from build123d import *

# Parameters (mm, degrees)
SKETCH1_R               = 7.5565
BOSS_EXTRUDE1_DEPTH     = 15.875
BOSS_EXTRUDE2_START     = 3.175
SKETCH2_R               = 7.5565
SKETCH2_R_2             = 3.3782
BOSS_EXTRUDE2_DEPTH     = 3.175
CUT_EXTRUDE1_DEPTH      = 20.136797263
CUT_EXTRUDE1_DEPTH_BACK = 20.136797263
SKETCH3_W               = 1.979009817
SKETCH3_H               = 3.81
SKETCH3_W_2             = 2.256055482


with BuildPart() as part:
    # Sketch1 → Boss-Extrude1 (new body)
    with BuildSketch(Plane(origin=(0, 0, 0), x_dir=(1, 0, 0), z_dir=(0, 1, 0))):
        with Locations(Location((0, 0, 0), (0, 0, 270))):
            Circle(SKETCH1_R)
        Polygon((-3.207902433, 5.55625), (-6.415804866, 0), (-3.207902433, -5.55625), (3.207902433, -5.55625), (6.415804866, 0), (3.207902433, 5.55625), align=None, mode=Mode.SUBTRACT)
    extrude(amount=BOSS_EXTRUDE1_DEPTH)

    # Sketch2 → Boss-Extrude2 (add)
    with BuildSketch(Plane.XZ.offset(BOSS_EXTRUDE2_START)):
        with Locations(Location((0, 0, 0), (0, 0, 270))):
            Circle(SKETCH2_R)
        with Locations(Location((0, 0, 0), (0, 0, 270))):
            Circle(SKETCH2_R_2, mode=Mode.SUBTRACT)
    extrude(amount=-BOSS_EXTRUDE2_DEPTH)

    # Sketch3 → Cut-Extrude1 (cut, two sides: drawn at the far end of the back side and taken through both)
    with BuildSketch(Plane(origin=(0, 0, 0), x_dir=(0, 0, -1), z_dir=(1, 0, 0)).offset(-CUT_EXTRUDE1_DEPTH_BACK)):
        with Locations((-7.212504909, 5.08)):
            Rectangle(SKETCH3_W, SKETCH3_H)
        with Locations((7.351027741, 5.08)):
            Rectangle(SKETCH3_W_2, SKETCH3_H)
    extrude(amount=CUT_EXTRUDE1_DEPTH + CUT_EXTRUDE1_DEPTH_BACK, mode=Mode.SUBTRACT)


solid = part.part
Work out the finished part from the listing and answer in its coordinate system (mm). A direction names the side the tool comes from. Give positions to 0.01 mm unless a question says otherwise; leave off trailing zeros. Order: outer loops, then holes, each group sorted by start corner. A loop starts at its lowest first (then second) coordinate and runs counter-clockwise, first axis right, second up. Notation, with made-up numbers: (57.25, -31) - (84.25, -31) arc R22 cw to (84.25, -25) - close; hole circle Ø10 at (13.5, 50.25). An arc over 180 degrees is marked (long way). Answer as CSV lines item,"result". Start each with the question number.
Q1. For faces 1 (the face through (-3.3, -1.61, 0.73)), 2 (the face through (4.834, 7.826, -2.739)), 3 (the face through (0, 6.985, -7)), 4 (the face through (0, 5, 6.223)), determine the directions among +Z, -Z, +X, -X, +Y, -Y from which every point of the face is accessible in a straight line to the end or side of a thin tool.
Q2. The part is cut by section B-B (x = 0). Write down the section's boundary in (y, z) (1 decimal), then the cut area to 3 significant figures.
Q3. Find the intervals of material crossed by L1, parallel to X at y = -1.75, z = 0; L2, parallel to Y at x = 3.25, z = -2.5 (3 decimals); L3, parallel to X at y = 3.25, z = 5, in increasing order. Write a range as [from, to].
Q4. The mould has two halves that part along Y. Classify faces 5 (the face through (0, 6.985, 7)), 6 (the face through (0, 15.875, 6)), 7 (the face through (-2, -3.175, -3)), 8 (the face through (4.8, 7.8, 2.8)): +Y half, -Y half, draft (parallel to the pull), parting line (faces both ways), or undercut.
Q5. The part is cut by section A-A (y = 0.75). Write down the section's boundary in (x, z).
Q6. Given pin 1 Ø1.9 at (x, y) = (0, 4.5) entering from +Z; pin 2 Ø3 at (x, y) = (-4, 11.5) entering from -Z; pin 3 Ø5 at (x, y) = (4.5, -0.5) entering from +Z; pin 4 Ø5.5 at (x, z) = (0, 0) entering from +Y, each flat-ended and moving along its own axis, determine where each tip first touches the part or whether it passes through.
Q7. The part is cut by section C-C (z = 6.5). Write down the section's boundary in (x, y) (3 decimals).
Q8. The part is cut by section D-D (y = 3.5). Write down the section's boundary in (x, z), then the cut area to 3 significant figures.
Check result:
1,face 1,"+Y, -Y"
1,face 2,"+Y"
1,face 3,"-Z, +X, -X"
1,face 4,"+Z, +X, -X"
2,outline,"(-3.2, -7.6) - (3.2, -7.6) - (3.2, -6.2) - (7, -6.2) - (7, -7.6) - (15.9, -7.6) - (15.9, -5.6) - (0, -5.6) - (0, -3.4) - (-3.2, -3.4) - close; (-3.2, 3.4) - (0, 3.4) - (0, 5.6) - (15.9, 5.6) - (15.9, 7.6) - (7, 7.6) - (7, 6.2) - (3.2, 6.2) - (3.2, 7.6) - (-3.2, 7.6) - close"
2,area,"79.9 mm²"
3,L1,"x = [-7.56, -3.38], [3.38, 7.56]"
3,L2,"y = [-3.175, 0]"
3,L3,"x = [-5.67, -3.53], [3.53, 5.67]"
4,face 5,"undercut"
4,face 6,"+Y half"
4,face 7,"-Y half"
4,face 8,"draft"
5,outline,"circle Ø15.11 at (0, 0); hole (-6.42, 0) - (-3.21, -5.56) - (3.21, -5.56) - (6.42, 0) - (3.21, 5.56) - (-3.21, 5.56) - close"
6,pin 1,"stops at z = 6.22"
6,pin 2,"stops at z = -7.13"
6,pin 3,"stops at z = 7.29"
6,pin 4,"passes through"
7,outline,"(-3.854, -3.175) - (3.854, -3.175) - (3.854, 3.175) - (-3.854, 3.175) - close; (-3.854, 6.985) - (3.854, 6.985) - (3.854, 15.875) - (-3.854, 15.875) - close"
8,outline,"(-4.29, -6.22) - (4.29, -6.22) arc R7.56 ccw to (4.29, 6.22) - (-4.29, 6.22) arc R7.56 ccw to start; hole (-6.42, 0) - (-3.21, -5.56) - (3.21, -5.56) - (6.42, 0) - (3.21, 5.56) - (-3.21, 5.56) - close"
8,area,"56.9 mm²"
